Autodesk Inventor part; units mm, degrees
ref_plane "YZ Plane" through (0, 0, 0) normal (1, 0, 0) x (0, 1, 0)
ref_plane "XZ Plane" through (0, 0, 0) normal (0, 1, 0) x (-1, 0, 0)
ref_plane "XY Plane" through (0, 0, 0) normal (0, 0, 1) x (1, 0, 0)
sketch "Sketch1" plane through (0, 0, 0) normal (0, 0, 1) x (1, 0, 0)
  line L0 (-11.9586, 8.8362) -> (0.7914, 8.8362)
  line L1 (0.7914, 8.8362) -> (0.7914, -5.1638)
  line L2 (0.7914, -5.1638) -> (-11.9586, -5.1638)
  line L3 (-11.9586, -5.1638) -> (-11.9586, 8.8362)
  circle A0 centre (-5.5836, 1.8362) radius 4.2944
  dimension "d0" = 12.75
  dimension "d1" = 14
  dimension "d2" = 6.375
  dimension "d3" = 7
extrude "Extrusion1" add sketch "Sketch1" along normal blind 12
sketch "Sketch2" plane through (0, 0, 12) normal (0, 0, 1) x (1, 0, 0)
  line L0 (0.7914, 8.8362) -> (0.7914, -5.1638)
  line L1 (-11.9586, 8.8362) -> (0.7914, 8.8362)
  line L2 (-11.9586, -5.1638) -> (-11.9586, 8.8362)
  line L3 (-11.9586, 6.3362) -> (0.7914, 6.3362)
  dimension "d7" = 2.5
extrude "Extrusion2" add sketch "Sketch2" along normal blind 17.5
sketch "Sketch3" plane through (-11.9586, 6.3362, 12) normal (0, -1, 0) x (1, 0, 0)
  line L0 (12.75, 17.5) -> (0, 17.5)
  line L1 (0, 0) -> (0, 17.5)
  point P0 (6.375, 9.5)
  dimension "d10" = 8
  dimension "d11" = 6.375
hole "Hole1" at (-5.5836, 6.3362, 21.5) direction (0, 1, 0) diameter 6.5 end through all
sketch "Sketch4" plane through (-11.9586, -5.1638, 0) normal (0, -1, 0) x (1, 0, 0)
  line L0 (12.75, 12) -> (0, 12)
  line L1 (0, 0) -> (0, 12)
  point P0 (6.375, 6)
  dimension "d19" = 6.375
  dimension "d20" = 6
hole "Hole2" at (-5.5836, -5.1638, 6) direction (0, 1, 0) diameter 6.917 depth 7 tip angle 118
equation "\"d2\" = 0.5 * d0"
equation "\"d3\" = 0.5 * d1"
properties part number "Terminal Battery" material "Copper"
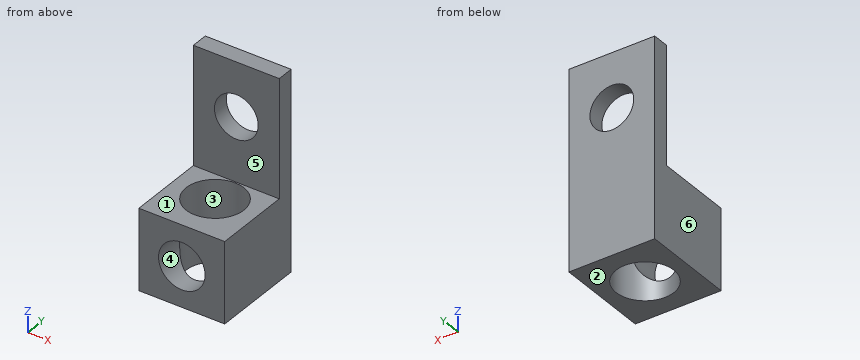
Verification items for the finished model (mm, model axes). Face numbers are marked on the shaded views. A direction names the side the tool comes from. Coordinates: 2 decimals unless noted, no trailing zeros. Loops run counter-clockwise (first coordinate to the right, second up) from the corner with the lowest first, then second, coordinate; pieces in that order, holes last. Notation, with made-up numbers: (23, 19) - (76, 19) arc R28 ccw to (76, 44) - close; hole circle Ø5 at (-3, 49.25). An arc over 180 degrees is marked (long way). Put each result on its own line as item: value.
Item 1: Section check A-A (z = 21.5). Enter the section's corners in (x, y), then the cut area to 3 significant figures.
Conclusion:
outline: (-11.96, 6.34) - (-8.83, 6.34) - (-8.83, 8.84) - (-11.96, 8.84) - close; (-2.33, 6.34) - (0.79, 6.34) - (0.79, 8.84) - (-2.33, 8.84) - close
area: 15.6 mm2
Item 2: Section check C-C (x = -4). Enter the section's corners in (y, z), then the cut area to 3 significant figures.
Conclusion:
outline: (-5.16, 0) - (-2.16, 0) - (-2.16, 2.93) - (-5.16, 2.93) - close; (-5.16, 9.07) - (-2.16, 9.07) - (-2.16, 12) - (-5.16, 12) - close; (5.83, 0) - (8.84, 0) - (8.84, 18.66) - (6.34, 18.66) - (6.34, 12) - (5.83, 12) - close; (6.34, 24.34) - (8.84, 24.34) - (8.84, 29.5) - (6.34, 29.5) - close
area: 83.3 mm2
Item 3: Gauge pin test, flat end, axial feed: pin 1 Ø4 at (x, z) = (-7, 23.5) entering from -Y. Record the tip position at first contact, or that the pin passes through.
Conclusion:
pin 1: stops at y = 6.34
Item 4: Section check B-B (y = -1.75). Enter the section's corners in (x, z), then the cut area to 3 significant figures.
Conclusion:
outline: (-11.96, 0) - (-7.95, 0) - (-7.95, 3.47) arc R3.46 cw to (-7.95, 8.53) - (-7.95, 12) - (-11.96, 12) - close; (-3.22, 0) - (0.79, 0) - (0.79, 12) - (-3.22, 12) - (-3.22, 8.53) arc R3.46 cw to (-3.22, 3.47) - close
area: 88.6 mm2
Item 5: Section check D-D (z = 6). Enter the section's corners in (x, y), then the cut area to 3 significant figures.
Conclusion:
outline: (-11.96, -5.16) - (-9.04, -5.16) - (-9.04, -0.71) arc R4.29 cw (long way) to (-2.13, -0.71) - (-2.13, -5.16) - (0.79, -5.16) - (0.79, 8.84) - (-11.96, 8.84) - close
area: 98.2 mm2
Item 6: Set-up check for the marked faces 1 and 2: record each of +Z, -Z, +X, -X, +Y, -Y from which the full face is reachable in a straight line by a thin tool's end or side.
Conclusion:
face 1: +Z, +X, -X, -Y
face 2: -Z, +X, -X, +Y, -Y
Item 7: Scan lines: line 1 along X through (y, z) = (6.5, 21.5); line 2 along X through (y, z) = (-2.1, 6); line 3 along Z through (x, y) = (-10.5, 2). Record each from-to range of solid material in increasing order.
Conclusion:
line 1: x = -11.96 to -8.83, -2.33 to 0.79
line 2: x = -11.96 to -9.04, -2.13 to 0.79
line 3: z = 0 to 12
Item 8: Draft check along X on the marked faces 3, 4, 5 and 6. Enter one of: pulls with the +X half, pulls with the -X half, needs draft (parallel to the pull), parting line crosses it, or undercut.
Conclusion:
face 3: undercut
face 4: undercut
face 5: needs draft
face 6: pulls with the -X half
